Geometry check sheet. Reference: the model listing, model coordinates, mm. A direction names the side the tool comes from. Round coordinates to 2 decimals unless told otherwise and drop trailing zeros. Write each loop counter-clockwise with the first axis right and the second up, starting at its lowest first coordinate (ties: lowest second). Pieces come first, ordered by that corner, then holes. Notation, with made-up numbers: (-7.5, 18) - (0.5, 18) arc R15 cw to (0.5, 41) - close; hole circle Ø7 at (78, 41.5). An arc over 180 degrees is marked (long way). Return JSON: item names as keys, results as strings. Group by question number.
from build123d import *

# Parameters (mm, degrees)
F3_DEPTH = 0.2
F4_COUNT = 4


# Not quite as in the source:
# - a feature names something its author has since deleted; it is built from what else it names


with BuildPart() as f1:
    # F0 (on Front) → F1 (revolve)
    with BuildSketch(Plane.XZ):
        with BuildLine():
            Line((0, 14.0277777778), (0, 0))
            Line((0, 0), (0.5555555556, 0))
            Line((0.5555555556, 0), (0.5555555556, 12.3611111111))
            ThreePointArc((0.5555555556, 12.3611111111), (0.5078793667, 13.0620116793), (0.3657291084, 13.75))
            ThreePointArc((0.3657291084, 13.75), (0.2296291982, 13.9504603784), (0, 14.0277777778))
        make_face()
    revolve(axis=Axis((0, 0, 7.0138888889), (0, 0, 1)))

    # F2 (on Front) → F3 (join, symmetric)
    with BuildSketch(Plane.XZ):
        with BuildLine():
            Line((0, 12.6567901235), (0, 0.6944444444))
            Line((0, 0.6944444444), (2.1180555556, 0.6944444444))
            Line((2.1180555556, 0.6944444444), (2.1180555556, 1.5277777778))
            Line((2.1180555556, 1.5277777778), (1.7534722222, 1.5277777778))
            Line((1.7534722222, 1.5277777778), (1.6145833333, 1.5277777778))
            Line((1.6145833333, 1.5277777778), (0.4, 1.5277777778))
            Line((0.4, 1.5277777778), (0.4, 1.875))
            Line((0.4, 1.875), (1.5972222222, 1.875))
            Line((1.5972222222, 1.875), (1.7708333333, 1.875))
            Line((1.7708333333, 1.875), (2.1180555556, 1.875))
            Line((2.1180555556, 1.875), (0.8333333333, 7.7624119633))
            ThreePointArc((0.8333333333, 7.7624119633), (0.7338823641, 7.9232334612), (0.5555555556, 7.9861111111))
            Line((0.5555555556, 7.9861111111), (0.2, 7.9861111111))
            Line((0.2, 7.9861111111), (0.2, 9.8947530864))
            Line((0.2, 9.8947530864), (0.8680555556, 11.5277777778))
            Line((0.8680555556, 11.5277777778), (0.8680555556, 11.8402777778))
            Line((0.8680555556, 11.8402777778), (0.2, 12.6567901235))
            Line((0.2, 12.6567901235), (0, 12.6567901235))
        make_face()
        Polygon((1.6145833333, 1.5277777778), (1.7534722222, 1.5277777778), (1.7708333333, 1.875), (1.5972222222, 1.875), align=None)
    extrude(amount=F3_DEPTH, both=True)

    # F4: F1 ×4 about axis
    f4_axis = Axis((0, 0, 0), (0, 0, 1))


with BuildPart() as f1_1:
    add(f1.part)
    for i in range(1, F4_COUNT):
        add(f1.part.rotate(f4_axis, i * 360 / F4_COUNT))


solid = f1_1.part
1. Section check C-C (y = 1.25). Enter the section's corners in (x, z) (3 decimals), and give its area (3 significant figures).
2. Tool access check on faces 4 (the face through (-1, 0.2, 4)), 5 (the face through (1, -0.2, 4)), 6 (the face through (0.2, 1, 4)), 7 (the face through (-0.2, -1, 4)). Record the directions out of +Z, -Z, +X, -X, +Y, -Y that give a thin tool (end or side, any length) a straight path to the whole face; none if there is none.
3. Section check D-D (z = 4.25). Enter the section's corners in (x, y).
4. Mould release check, pull along Z, two halves, no side actions. Record for faces 1 (the face through (-0.2, 1, 4)), 2 (the face through (0, 0, 0)), 3 (the face through (-0.44, -0.34, 6.27)): pulls with the +Z half, pulls with the -Z half, needs draft (parallel to the pull), parting line crosses it, or undercut.
5. Section check A-A (y = -0.7). Enter the section's corners in (x, z) (3 decimals), and give its area (3 significant figures).
6. Material ranges on line 1 along X through (y, z) = (0.65, 2); line 2 along X through (y, z) = (0.25, 10), recorded low to high.
7. Depth check by flat-ended pin: pin 1 Ø1.3 at (y, z) = (-1.5, 2.5) entering from +X. Enter the tip coordinate at first touch or a pass-through.
8. Section check B-B (x = 1.1). Enter the section's corners in (y, z) (3 decimals), and give its area (3 significant figures).
Result sheet:
{
 "1": {"outline": "(-0.2, 0.694) - (0.2, 0.694) - (0.2, 1.528) - (-0.2, 1.528) - close; (-0.2, 1.875) - (0.2, 1.875) - (0.2, 5.853) - (-0.2, 5.853) - close", "area": "1.92 mm²"},
 "2": {"face 4": "+Z, -Z, -X, +Y", "face 5": "+Z, -Z, +X, -Y", "face 6": "+Z, -Z, +X, +Y", "face 7": "+Z, -Z, -X, -Y"},
 "3": {"outline": "(-1.6, -0.2) - (-0.52, -0.2) arc R0.56 ccw to (-0.2, -0.52) - (-0.2, -1.6) - (0.2, -1.6) - (0.2, -0.52) arc R0.56 ccw to (0.52, -0.2) - (1.6, -0.2) - (1.6, 0.2) - (0.52, 0.2) arc R0.56 ccw to (0.2, 0.52) - (0.2, 1.6) - (-0.2, 1.6) - (-0.2, 0.52) arc R0.56 ccw to (-0.52, 0.2) - (-1.6, 0.2) - close"},
 "4": {"face 1": "needs draft", "face 2": "pulls with the -Z half", "face 3": "undercut"},
 "5": {"outline": "(-0.2, 0.694) - (0.2, 0.694) - (0.2, 1.528) - (-0.2, 1.528) - close; (-0.2, 1.875) - (0.2, 1.875) - (0.2, 7.947) - (-0.2, 7.947) - close; (-0.2, 11.117) - (0.2, 11.117) - (0.2, 12.046) - (-0.2, 12.046) - close", "area": "3.13 mm²"},
 "6": {"line 1": "x = -0.2 to 0.2", "line 2": "x = -0.5 to 0.5"},
 "7": {"pin 1": "stops at x = 0.2"},
 "8": {"outline": "(-0.2, 0.694) - (0.2, 0.694) - (0.2, 1.528) - (-0.2, 1.528) - close; (-0.2, 1.875) - (0.2, 1.875) - (0.2, 6.54) - (-0.2, 6.54) - close", "area": "2.20 mm²"}
}
